Check sheet for the modelled part. Datum: model origin and axes. Units: mm. Face numbers are marked on the shaded views. A direction names the side the tool comes from. Coordinates: 2 decimals unless noted, no trailing zeros. Loops run counter-clockwise (first coordinate to the right, second up) from the corner with the lowest first, then second, coordinate; pieces in that order, holes last. Notation, with made-up numbers: (-20, 14) - (-16, 14) arc R29 cw to (-16, 52) - close; hole circle Ø11 at (7.5, -39). An arc over 180 degrees is marked (long way). Use a Markdown table: item, result. Add a question column.
1) Draft check along Y on the marked faces 4, 5, 6 and 7. Enter one of: pulls with the +Y half, pulls with the -Y half, needs draft (parallel to the pull), parting line crosses it, or undercut.
2) Tool access check on the marked faces 1, 2 and 3. Record the directions out of +Z, -Z, +X, -X, +Y, -Y that give a thin tool (end or side, any length) a straight path to the whole face; none if there is none.
3) Sectioned sample at B-B, the plane z = -10. Enter the section's corners in (x, y), then the cut area to 3 significant figures.
4) Sectioned sample at C-C, the plane y = -45. Enter the section's corners in (x, z), then the cut area to 3 significant figures.
5) Sectioned sample at A-A, the plane x = 25. Enter the section's corners in (y, z).
6) Go/stop test with flat-tipped pins: P1, Ø8, axis at y = 41.5, z = 5.5, coming from the +X side; P2, Ø3, axis at x = 40, y = -30.5, coming from the +Z side; P3, Ø2, axis at y = 32, z = 0, coming from the +X side. Record where each tip stops, or that it passes through.
7) Thickness scan on line 1 (X direction, y = -3.5, z = -7.5); line 2 (X direction, y = -57, z = 0.5); line 3 (Z direction, x = 41, y = -18). Record the ranges inside material, lowest first.
8) Sectioned sample at D-D, the plane y = 39.5. Enter the section's corners in (x, z).
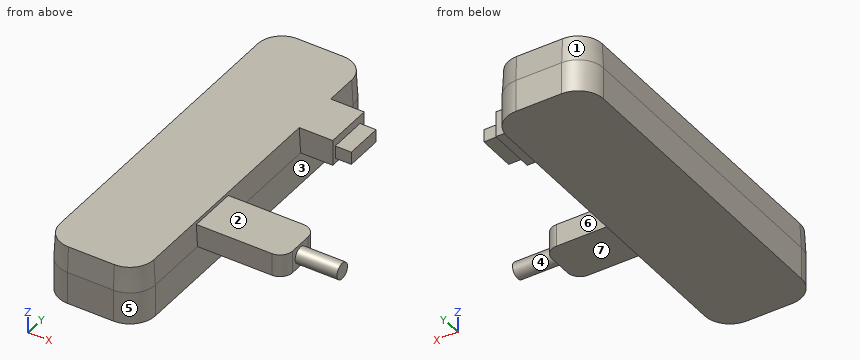
from build123d import *

# Parameters (mm, degrees)
F1_DEPTH      = 12.7
F1_DEPTH_BACK = 10.16
F1_TAPER_BACK = 3
F2_W          = 19.304
F2_H          = 8.89
F3_DEPTH      = 34.29
F3_DEPTH_BACK = 0.4659051578
F4_R          = 5
F5_R          = 3.175
F6_DEPTH      = 16.51
F7_W          = 19.05
F7_H          = 10.16
F8_DEPTH      = 12.7
F8_DEPTH_BACK = 0.5324630375
F9_W          = 15
F9_H          = 5
F10_DEPTH     = 6.35


with BuildPart() as f1:
    # F0 (on Top) → F1 (new body, two sides)
    with BuildSketch(Plane.XY) as f1_sk:
        with BuildLine():
            Line((9.05, 69.85), (-9.05, 69.85))
            ThreePointArc((-9.05, 69.85), (-16.1210678119, 66.9210678119), (-19.05, 59.85))
            Line((-19.05, 59.85), (-19.05, -59.85))
            ThreePointArc((-19.05, -59.85), (-16.1210678119, -66.9210678119), (-9.05, -69.85))
            Line((-9.05, -69.85), (9.05, -69.85))
            ThreePointArc((9.05, -69.85), (16.1210678119, -66.9210678119), (19.05, -59.85))
            Line((19.05, -59.85), (19.05, 59.85))
            ThreePointArc((19.05, 59.85), (16.1210678119, 66.9210678119), (9.05, 69.85))
        make_face()
    extrude(amount=-F1_DEPTH)
    extrude(f1_sk.sketch, amount=F1_DEPTH_BACK, taper=F1_TAPER_BACK)

    # F2 (on face) → F3 (join, two sides)
    with BuildSketch(Plane.YZ.offset(19.05)) as f3_sk:
        with Locations((-24.638, 4.445)):
            Rectangle(F2_W, F2_H)
    extrude(amount=F3_DEPTH)
    extrude(f3_sk.sketch, amount=-F3_DEPTH_BACK)

    # F4
    f4_edges = [f1.edges().sort_by_distance(p)[0] for p in [
        (53.34, -34.29, 4.445),
        (53.34, -14.986, 4.445),
    ]]
    fillet(f4_edges, radius=F4_R)

    # F5 (on face) → F6 (join)
    with BuildSketch(Plane.YZ.offset(53.34)):
        with Locations((-24.638, 4.445)):
            Circle(F5_R)
    extrude(amount=F6_DEPTH)

    # F7 (on face) → F8 (join, two sides)
    with BuildSketch(Plane.YZ.offset(19.05)) as f8_sk:
        with Locations((37.625, 5.08)):
            Rectangle(F7_W, F7_H)
    extrude(amount=F8_DEPTH)
    extrude(f8_sk.sketch, amount=-F8_DEPTH_BACK)

    # F9 (on face) → F10 (join)
    with BuildSketch(Plane.YZ.offset(31.75)):
        with Locations((37.1, 4.5)):
            Rectangle(F9_W, F9_H)
    extrude(amount=F10_DEPTH)


solid = f1.part
Solved:
| question | item | result |
|---|---|---|
| 1 | face 4 | parting line crosses it |
| 1 | face 5 | pulls with the -Y half |
| 1 | face 6 | undercut |
| 1 | face 7 | needs draft |
| 2 | face 1 | +Z, -X, +Y |
| 2 | face 2 | +Z, +X, -Y |
| 2 | face 3 | -Z, +X, +Y, -Y |
| 3 | outline | (-19.05, -59.85) arc R10 ccw to (-9.05, -69.85) - (9.05, -69.85) arc R10 ccw to (19.05, -59.85) - (19.05, 59.85) arc R10 ccw to (9.05, 69.85) - (-9.05, 69.85) arc R10 ccw to (-19.05, 59.85) - close |
| 3 | area | 5,240 mm2 |
| 4 | outline | (-19.05, -12.7) - (19.05, -12.7) - (19.05, 0) - (18.52, 10.16) - (-18.52, 10.16) - (-19.05, 0) - close |
| 4 | area | 866 mm2 |
| 5 | outline | (-34.29, 0) - (-14.99, 0) - (-14.99, 8.89) - (-34.29, 8.89) - close; (28.1, 0) - (47.15, 0) - (47.15, 10.16) - (28.1, 10.16) - close |
| 6 | P1 | stops at x = 38.1 |
| 6 | P2 | stops at z = 8.89 |
| 6 | P3 | stops at x = 31.75 |
| 7 | line 1 | x = -19.05 to 19.05 |
| 7 | line 2 | x = -19.02 to 19.02 |
| 7 | line 3 | z = 0 to 8.89 |
| 8 | outline | (-19.05, -12.7) - (19.05, -12.7) - (19.05, 0) - (31.75, 0) - (31.75, 2) - (38.1, 2) - (38.1, 7) - (31.75, 7) - (31.75, 10.16) - (-18.52, 10.16) - (-19.05, 0) - close |
